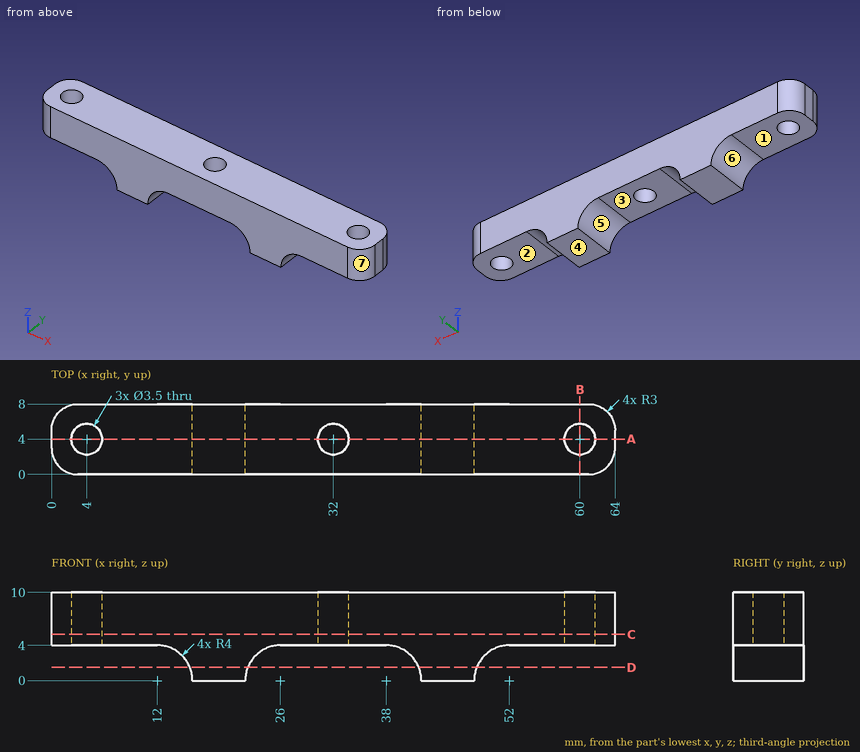
The drawing under review shows one solid part. Ordinate dimensions are in mm from its lowest x, y, z. A direction names the side the tool comes from. Give positions to 0.01 mm unless a question says otherwise; leave off trailing zeros. Order: outer loops, then holes, each group sorted by start corner. A loop starts at its lowest first (then second) coordinate and runs counter-clockwise, first axis right, second up. Notation, with made-up numbers: (9.25, 48.25) -> (37.25, 48.25) arc R20 ccw to (37.25, 63.25) -> close; hole circle Ø7 at (-38, -6.75). An arc over 180 degrees is marked (long way). Write item = value, one per line. Start each with the question number.
(1) To check wall thickness, follow line 1 along X through (y, z) = (4, 6.3); line 2 along Y through (x, z) = (32, 7.6); line 3 along X through (y, z) = (5.5, 4.5). State the ranges of each line that lie inside material, in increasing order.
(2) Mouldability with a two-part tool opening along X and no side actions: class the marked faces 4, 5, 6 and 7 as +X half, -X half, draft (parallel to the pull), parting line (faces both ways), or undercut.
(3) We need section D-D on z = 1.5. Write out the cut boundary in (x, y).
(4) We need section B-B on x = 60. Write out the cut boundary in (y, z), plus the area to 3 significant figures.
(5) We need section A-A on y = 4. Write out the cut boundary in (x, z).
(6) For pin 1 (4 mm diameter, centred on x = 57.5, y = 5, fed in from -Z), flat-tipped, find the tip position at first contact; note if it passes through.
(7) For the marked faces 1, 2 and 3, list the 3-axis set-ups (+Z, -Z, +X, -X, +Y, -Y) from which the entire face can be reached by the end or side of a thin tool; tool diameter is ignored.
(8) We need section C-C on z = 5.25. Write out the cut boundary in (x, y).
Numbers:
q1.line_1 = 0 to 2.25, 5.75 to 30.25, 33.75 to 58.25, 61.75 to 64
q1.line_2 = 0 to 2.25, 5.75 to 8
q1.line_3 = 0.04 to 3.1, 4.9 to 31.1, 32.9 to 59.1, 60.9 to 63.96
q2.face_4 = draft
q2.face_5 = undercut
q2.face_6 = -X half
q2.face_7 = +X half
q3.outline = (15.71, 0) -> (22.29, 0) -> (22.29, 8) -> (15.71, 8) -> close; (41.71, 0) -> (48.29, 0) -> (48.29, 8) -> (41.71, 8) -> close
q4.outline = (0, 4) -> (2.25, 4) -> (2.25, 10) -> (0, 10) -> close; (5.75, 4) -> (8, 4) -> (8, 10) -> (5.75, 10) -> close
q4.area = 27.0 mm^2
q5.outline = (0, 4) -> (2.25, 4) -> (2.25, 10) -> (0, 10) -> close; (5.75, 4) -> (12, 4) arc R4 cw to (16, 0) -> (22, 0) arc R4 cw to (26, 4) -> (30.25, 4) -> (30.25, 10) -> (5.75, 10) -> close; (33.75, 4) -> (38, 4) arc R4 cw to (42, 0) -> (48, 0) arc R4 cw to (52, 4) -> (58.25, 4) -> (58.25, 10) -> (33.75, 10) -> close; (61.75, 4) -> (64, 4) -> (64, 10) -> (61.75, 10) -> close
q6.pin_1 = 4
q7.face_1 = -Z, -X, +Y, -Y
q7.face_2 = -Z, +X, +Y, -Y
q7.face_3 = -Z, +Y, -Y
q8.outline = (0, 3) arc R3 ccw to (3, 0) -> (61, 0) arc R3 ccw to (64, 3) -> (64, 5) arc R3 ccw to (61, 8) -> (3, 8) arc R3 ccw to (0, 5) -> close; hole circle Ø3.5 at (4, 4); hole circle Ø3.5 at (32, 4); hole circle Ø3.5 at (60, 4)
